```python
from build123d import *

# Parameters (mm, degrees)
BOSS_EXTRUDE1_DEPTH   = 0.5
FILLET3_R             = 2
FILLET4_R             = 0.75
FILLET5_R             = 0.75
SKETCH2_W             = 0.5
SKETCH2_H             = 3
BOSS_EXTRUDE2_DEPTH   = 7.070737889
FILLET3_OF_MIRROR5_R  = 2
FILLET4_OF_MIRROR5_R  = 0.75
FILLET5_OF_MIRROR5_R  = 0.75
FILLET7_R             = 0.5
F_4_0MM_DOWEL_HOLE1_D = 4


with BuildPart() as part:
    # Sketch1 → Boss-Extrude1 (new body)
    with BuildSketch(Plane(origin=(0, 0, 0), x_dir=(1, 0, 0), z_dir=(0, 1, 0))):
        with BuildLine():
            Line((23.293714059, 86.933324366), (18.816144579, 70.222807571))
            Line((18.816144579, 70.222807571), (20.261027783, 69.819630142))
            Line((20.261027783, 69.819630142), (25.127648951, 87.982107603))
            ThreePointArc((25.127648951, 87.982107603), (14.434923875, 90.354208384), (3.535368944, 91.431674853))
            Line((3.535368944, 91.431674853), (3.535368944, 99))
            Line((3.535368944, 99), (-3.535368944, 99))
            Line((-3.535368944, 99), (-3.535368944, 91.431674853))
            ThreePointArc((-3.535368944, 91.431674853), (-14.434923875, 90.354208384), (-25.127648951, 87.982107603))
            Line((-25.127648951, 87.982107603), (-20.261027783, 69.819630142))
            Line((-20.261027783, 69.819630142), (-18.816144579, 70.222807571))
            Line((-18.816144579, 70.222807571), (-23.293714059, 86.933324366))
            ThreePointArc((-23.293714059, 86.933324366), (0, 90), (23.293714059, 86.933324366))
        make_face()
    boss_extrude1 = extrude(amount=BOSS_EXTRUDE1_DEPTH)

    # Fillet3
    fillet3_edges = [part.edges().sort_by_distance(p)[0] for p in [
        (-23.293714059, 0.25, -86.933324366),
        (-25.127648951, 0.25, -87.982107603),
        (25.127648951, 0.25, -87.982107603),
        (23.293714059, 0.25, -86.933324366),
    ]]
    fillet(fillet3_edges, radius=FILLET3_R)

    # Fillet4
    fillet4_edges = [part.edges().sort_by_distance(p)[0] for p in [
        (-18.816144579, 0.25, -70.222807571),
        (-20.261027783, 0.25, -69.819630142),
    ]]
    fillet(fillet4_edges, radius=FILLET4_R - 0.0001)  # a hair under: the kernel refuses the full size

    # Fillet5
    fillet5_edges = [part.edges().sort_by_distance(p)[0] for p in [
        (20.261027783, 0.25, -69.819630142),
        (18.816144579, 0.25, -70.222807571),
    ]]
    fillet(fillet5_edges, radius=FILLET5_R - 0.0001)  # a hair under: the kernel refuses the full size

    # Sketch2 → Boss-Extrude2 (add)
    with BuildSketch(Plane(origin=(3.535368944, 0, 0), x_dir=(0, 0, -1), z_dir=(1, 0, 0))):
        with Locations((99.25, 1.5)):
            Rectangle(SKETCH2_W, SKETCH2_H)
    boss_extrude2 = extrude(amount=-BOSS_EXTRUDE2_DEPTH)

    # Mirror3: Boss-Extrude2 across plane
    add(boss_extrude2.mirror(Plane.ZX.offset(3)))

    # Mirror5: Boss-Extrude1 across plane
    add(boss_extrude1.mirror(Plane.ZX.offset(3)))

    # Fillet3 of Mirror5
    fillet3_of_mirror5_edges = [part.edges().sort_by_distance(p)[0] for p in [
        (-23.293714059, 5.75, -86.933324366),
        (-25.127648951, 5.75, -87.982107603),
        (25.127648951, 5.75, -87.982107603),
        (23.293714059, 5.75, -86.933324366),
    ]]
    fillet(fillet3_of_mirror5_edges, radius=FILLET3_OF_MIRROR5_R)

    # Fillet4 of Mirror5
    fillet4_of_mirror5_edges = [part.edges().sort_by_distance(p)[0] for p in [
        (-18.816144579, 5.75, -70.222807571),
        (-20.261027783, 5.75, -69.819630142),
    ]]
    fillet(fillet4_of_mirror5_edges, radius=FILLET4_OF_MIRROR5_R - 0.0001)  # a hair under: the kernel refuses the full size

    # Fillet5 of Mirror5
    fillet5_of_mirror5_edges = [part.edges().sort_by_distance(p)[0] for p in [
        (20.261027783, 5.75, -69.819630142),
        (18.816144579, 5.75, -70.222807571),
    ]]
    fillet(fillet5_of_mirror5_edges, radius=FILLET5_OF_MIRROR5_R - 0.0001)  # a hair under: the kernel refuses the full size

    # Fillet7
    fillet7_edges = [part.edges().sort_by_distance(p)[0] for p in [
        (0, 5.5, -99),
        (0, 0.5, -99),
        (0, 0, -99.5),
        (0, 6, -99.5),
    ]]
    fillet(fillet7_edges, radius=FILLET7_R)

    # Ø4.0mm Dowel Hole1 (through all)
    with Locations(Plane(origin=(0, 6, 0), x_dir=(1, 0, 0), z_dir=(0, 1, 0))):
        with Locations((0, 96.5)):
            Hole(F_4_0MM_DOWEL_HOLE1_D / 2)


solid = part.part
```
Check sheet for the modelled part. Datum: model origin and axes. Units: mm. A direction names the side the tool comes from. Give positions to 0.01 mm unless a question says otherwise; leave off trailing zeros. Order: outer loops, then holes, each group sorted by start corner. A loop starts at its lowest first (then second) coordinate and runs counter-clockwise, first axis right, second up. Notation, with made-up numbers: M 74.5,-40 L 98.5,-40 A9 cw 98.5,-29 Z; hole C 22,72 d7. An arc over 180 degrees is marked long. Answer in a Markdown table with one row per item.
1) Access from +Z, -Z, +X, -X, +Y, -Y to the whole of each face (thin tool, end or side, straight path). Record for faces 1 (the flat face through (0, 5.5, -91)), 2 (the flat face through (-20.863, 5.754, -77.861)), 3 (the cylindrical face through (24.4, 0.3, -87.6)).
Filled sheet:
| item | result |
|---|---|
| face 1 | +Z, +X, -X |
| face 2 | +Y, -Y |
| face 3 | +X, +Y, -Y |
2) Cross-section at B-B, the plane z = -96.5. Enter the section's corners in (x, y), plus the area to 3 significant figures.
Filled sheet:
| item | result |
|---|---|
| outline | M -3.54,0 L -2,0 L -2,0.5 L -3.54,0.5 Z; M -3.54,5.5 L -2,5.5 L -2,6 L -3.54,6 Z; M 2,0 L 3.54,0 L 3.54,0.5 L 2,0.5 Z; M 2,5.5 L 3.54,5.5 L 3.54,6 L 2,6 Z |
| area | 3.07 mm2 |
3) Cross-section at C-C, the plane x = 8.5. Enter the section's corners in (y, z).
Filled sheet:
| item | result |
|---|---|
| outline | M 0,-91.1 L 0.5,-91.1 L 0.5,-89.6 L 0,-89.6 Z; M 5.5,-91.1 L 6,-91.1 L 6,-89.6 L 5.5,-89.6 Z |
4) Release check for a two-part mould opening along Z. For faces 4 (the cylindrical face through (-13.3, 5.75, -90.53)), 5 (the cylindrical face through (0.26, 5.746, -98.483)), 6 (the flat face through (-22.564, 0.246, -78.415)) record: +Z half, -Z half, draft (parallel to the pull), parting line (faces both ways), or undercut.
Filled sheet:
| item | result |
|---|---|
| face 4 | -Z half |
| face 5 | undercut |
| face 6 | +Z half |
5) Cross-section at A-A, the plane x = -16.5. Enter the section's corners in (y, z), plus the area to 3 significant figures.
Filled sheet:
| item | result |
|---|---|
| outline | M 0,-90 L 0.5,-90 L 0.5,-88.47 L 0,-88.47 Z; M 5.5,-90 L 6,-90 L 6,-88.47 L 5.5,-88.47 Z |
| area | 1.53 mm2 |
6) Gauge pin test, flat ends, axial feed: P1, Ø8, axis at x = -13, z = -88.5, coming from the -Y side; P2, Ø2, axis at x = -17.5, y = 1, coming from the +Z side. Record the tip position at first contact, or that the pin passes through.
Filled sheet:
| item | result |
|---|---|
| P1 | stops at y = 0 |
| P2 | stops at z = -88.11 |
7) Cross-section at D-D, the plane y = 2.5. Enter the section's corners in (x, z).
Filled sheet:
| item | result |
|---|---|
| outline | M -3.54,-99.5 L 3.54,-99.5 L 3.54,-99 L -3.54,-99 Z |
8) Thickness scan on L1, parallel to X at y = 5.7, z = -96.5; L2, parallel to Y at x = 22, z = -87.25; L3, parallel to Z at x = -2, y = 2.15. Record the ranges inside material, lowest first. Write a range as [from, to].
Filled sheet:
| item | result |
|---|---|
| L1 | x = [-3.54, -2], [2, 3.54] |
| L2 | y = [0, 0.5], [5.5, 6] |
| L3 | z = [-99.5, -99] |
